from build123d import *

# Parameters (mm, degrees)
SKETCH1_W           = 29
SKETCH1_H           = 29
BOSS_EXTRUDE1_DEPTH = 0.4
SKETCH2_W           = 24.5
SKETCH2_H           = 24.5
SKETCH2_W_2         = 16
SKETCH2_H_2         = 16
BOSS_EXTRUDE2_DEPTH = 0.3
FILLET1_R           = 5
FILLET2_R           = 1


with BuildPart() as part:
    # Sketch1 → Boss-Extrude1 (new body)
    with BuildSketch(Plane.XY):
        with Locations((14.5, 14.5)):
            Rectangle(SKETCH1_W, SKETCH1_H)
    extrude(amount=BOSS_EXTRUDE1_DEPTH)

    # Sketch2 → Boss-Extrude2 (add)
    with BuildSketch(Plane.XY.offset(0.4)):
        with Locations((14.5, 14.5)):
            Rectangle(SKETCH2_W, SKETCH2_H)
        with Locations((14.5, 14.5)):
            Rectangle(SKETCH2_W_2, SKETCH2_H_2, mode=Mode.SUBTRACT)
    extrude(amount=BOSS_EXTRUDE2_DEPTH)

    # Fillet1
    fillet1_edges = [part.edges().sort_by_distance(p)[0] for p in [
        (2.25, 26.75, 0.55),
        (2.25, 2.25, 0.55),
        (26.75, 2.25, 0.55),
        (26.75, 26.75, 0.55),
    ]]
    fillet(fillet1_edges, radius=FILLET1_R)

    # Fillet2
    fillet2_edges = [part.edges().sort_by_distance(p)[0] for p in [
        (6.5, 6.5, 0.55),
        (22.5, 6.5, 0.55),
        (22.5, 22.5, 0.55),
        (6.5, 22.5, 0.55),
    ]]
    fillet(fillet2_edges, radius=FILLET2_R)


solid = part.part
Read the model definition and answer for the solid it produces. Units are mm, in the model's axes. A direction names the side the tool comes from. Give positions to 0.01 mm unless a question says otherwise; leave off trailing zeros. Loops run counter-clockwise (first coordinate to the right, second up) from the corner with the lowest first, then second, coordinate; pieces in that order, holes last. Notation, with made-up numbers: M 2.5,69 L 50.5,69 A26 ccw 50.5,105 Z; hole C 17.25,63.5 d2. An arc over 180 degrees is marked long. Write each question's results on one line, items separated by ' | '.
1. A tool of negligible diameter and unlimited length cuts with its end or side. For faces 3 (the face through (6, 15, 0.7)), 4 (the face through (1, 15, 0.4)), from which of +Z, -Z, +X, -X, +Y, -Y can it reach the whole face along a straight path? Write none if from no direction.
Values:
face 3: +Z, +X, -X, +Y, -Y | face 4: +Z
2. Given pin 1 (5 mm diameter, centred on x = 16, y = 12, fed in from +Z), flat-ended and moving along its own axis, determine where the tip first touches the part or whether it passes through.
Values:
pin 1: stops at z = 0.4
3. Section D-D on y = 26 is taken. Give the vertices of the cut face in (x, z), plus the area to 3 significant figures.
Values:
outline: M 0,0 L 29,0 L 29,0.4 L 24.38,0.4 L 24.38,0.7 L 4.62,0.7 L 4.62,0.4 L 0,0.4 Z | area: 17.5 mm^2
4. The mould has two halves that part along X. Classify faces 1 (the face through (14, 15, 0)), 2 (the face through (14, 15, 0.4)): pulls with the +X half, pulls with the -X half, needs draft (parallel to the pull), parting line crosses it, or undercut.
Values:
face 1: needs draft | face 2: undercut
5. Section C-C on x = 24.75 is taken. Give the vertices of the cut face in (y, z).
Values:
outline: M 0,0 L 29,0 L 29,0.4 L 25.75,0.4 L 25.75,0.7 L 3.25,0.7 L 3.25,0.4 L 0,0.4 Z
6. Straight lines are drawn through the part: line 1 (X direction, y = 13.5, z = 0.55); line 2 (Z direction, x = 15.25, y = 14.75). For each, find the intervals that lie inside material, in ascending order. Write a range as [from, to].
Values:
line 1: x = [2.25, 6.5], [22.5, 26.75] | line 2: z = [0, 0.4]
7. Section A-A on x = 18 is taken. Give the vertices of the cut face in (y, z).
Values:
outline: M 0,0 L 29,0 L 29,0.4 L 26.75,0.4 L 26.75,0.7 L 22.5,0.7 L 22.5,0.4 L 6.5,0.4 L 6.5,0.7 L 2.25,0.7 L 2.25,0.4 L 0,0.4 Z
